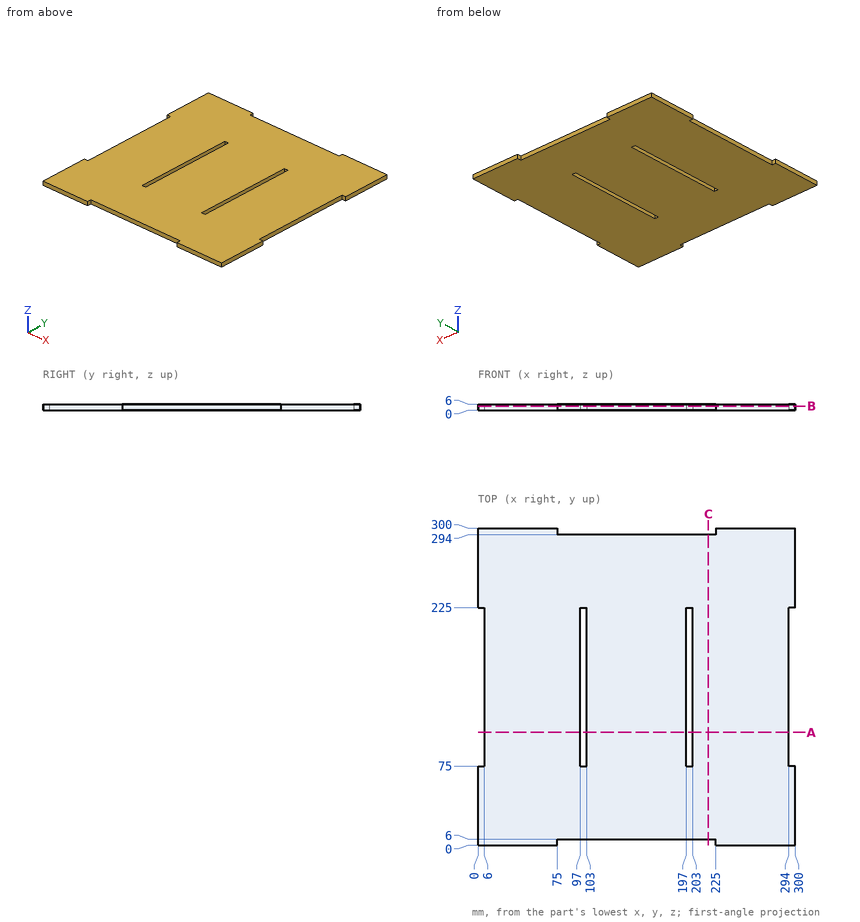
Drawing for the job (mm, zero at the part's lowest x, y, z). Give positions to 0.01 mm unless a question says otherwise; leave off trailing zeros. Loops run counter-clockwise (first coordinate to the right, second up) from the corner with the lowest first, then second, coordinate; pieces in that order, holes last. Notation, with made-up numbers: M 11,14 L 31,14 A14 ccw 31,37 Z; hole C -4,81.5 d6. An arc over 180 degrees is marked long. Use one line per item in the form item = value.
Item 1: Slice it at A-A (y = 107). List the corners of the cut face in (x, z), plus the area to 3 significant figures.
Determined:
outline = M 6,0 L 97,0 L 97,6 L 6,6 Z; M 103,0 L 197,0 L 197,6 L 103,6 Z; M 203,0 L 294,0 L 294,6 L 203,6 Z
area = 1,660 mm2
Item 2: Flat gauge pins, fed straight in: pin 1 (1 mm diameter, centred on y = 92.5, z = 1.5, fed in from -X); pin 2 (3 mm diameter, centred on y = 140.5, z = 3, fed in from +X); pin 3 (3 mm diameter, centred on x = 200.5, z = 2, fed in from +Y). Where does each tip first touch, or does it go through?
Determined:
pin_1 = 6
pin_2 = 294
pin_3 = 294
Item 3: Slice it at B-B (z = 3.9). List the corners of the cut face in (x, y), plus the area to 3 significant figures.
Determined:
outline = M 0,0 L 75,0 L 75,6 L 225,6 L 225,0 L 300,0 L 300,75 L 294,75 L 294,225 L 300,225 L 300,300 L 225,300 L 225,294 L 75,294 L 75,300 L 0,300 L 0,225 L 6,225 L 6,75 L 0,75 Z; hole M 97,75 L 103,75 L 103,225 L 97,225 Z; hole M 197,75 L 203,75 L 203,225 L 197,225 Z
area = 84,600 mm2
Item 4: Slice it at C-C (x = 218). List the corners of the cut face in (y, z).
Determined:
outline = M 6,0 L 294,0 L 294,6 L 6,6 Z
Item 5: Drill centre lines: probe 1 along X at (y, z) = (203, 3.85); probe 2 along Y at (x, z) = (101.5, 5.35); probe 3 along Y at (x, z) = (186.5, 1.2). Where is each one in solid material? Low to high. Write a range as from..to.
Determined:
probe_1 = 6..97, 103..197, 203..294
probe_2 = 6..75, 225..294
probe_3 = 6..294
